Work out the finished part from the listing and answer in its coordinate system (mm). A direction names the side the tool comes from. Coordinates: 2 decimals unless noted, no trailing zeros. Order: outer loops, then holes, each group sorted by start corner. A loop starts at its lowest first (then second) coordinate and runs counter-clockwise, first axis right, second up. Notation, with made-up numbers: M 84.25,78.5 L 140.25,78.5 A25 cw 140.25,90.5 Z; hole C -27,-3.5 d8. An arc over 180 degrees is marked long. Answer in a Markdown table with one row per item. Add a question column.
Item 1: Which of the six approach directions +Z, -Z, +X, -X, +Y, -Y give full straight-line access (tool end or side, diameter ignored) to faces 1 (the face through (69, -44, 0.254)), 2 (the face through (69, -88.9, 8))?
Item 2: The part is cut by section A-A (z = 2.75). Write down the section's boundary in (x, y).
Item 3: Consider line 1 (Z direction, x = 99, y = -11); line 2 (X direction, y = -35.5, z = 4.75); line 3 (X direction, y = -69.5, z = 13). Determine where each line is inside the solid, lowest interval first. Write a range as from..to.
Item 4: The part is cut by section C-C (y = -20.5). Write down the section's boundary in (x, z).
Item 5: Flat-ended cylindrical pins translate along their axes: pin 1 Ø1 at (y, z) = (-40.5, 8) entering from -X; pin 2 Ø1.5 at (y, z) = (-75.5, 12) entering from -X; pin 3 Ø3 at (x, z) = (123, 5) entering from -Y. Find the tip coordinate at first contact, or state that the pin passes through.
Item 6: The mould has two halves that part along X. Classify faces 3 (the face through (69, -88.646, 8)), 4 (the face through (69, -44, 0)): released by +X, released by -X, zero draft, split by the parting line, or undercut.
Item 7: The part is cut by section B-B (x = 47.5). Write down the section's boundary in (y, z).
from build123d import *

# Parameters (mm, degrees)
F1_DEPTH = 16.51
F2_T     = -0.254


with BuildPart() as f1:
    # F0 (on Top) → F1 (new body)
    with BuildSketch(Plane.XY):
        with BuildLine():
            Line((95.25, 0), (44.45, 0))
            ThreePointArc((44.45, 0), (13.019104, -13.019104), (0, -44.45))
            ThreePointArc((0, -44.45), (13.019104, -75.880896), (44.45, -88.9))
            Line((44.45, -88.9), (95.25, -88.9))
            ThreePointArc((95.25, -88.9), (126.680896, -75.880896), (139.7, -44.45))
            ThreePointArc((139.7, -44.45), (126.680896, -13.019104), (95.25, 0))
        make_face()
    extrude(amount=F1_DEPTH)

    # F2
    f2_openings = [f1.faces().sort_by_distance(p)[0] for p in [
        (69.85, -44.45, 16.51),
    ]]
    offset(amount=F2_T, openings=f2_openings)


solid = f1.part
Reply:
| question | item | result |
|---|---|---|
| 1 | face 1 | +Z |
| 1 | face 2 | +Z, -Z, +X, -X, -Y |
| 2 | outline | M 0,-44.45 A44.45 ccw 44.45,-88.9 L 95.25,-88.9 A44.45 ccw 139.7,-44.45 A44.45 ccw 95.25,0 L 44.45,0 A44.45 ccw Z; hole M 0.25,-44.45 A44.2 ccw 44.45,-88.65 L 95.25,-88.65 A44.2 ccw 139.45,-44.45 A44.2 ccw 95.25,-0.25 L 44.45,-0.25 A44.2 ccw Z |
| 3 | line 1 | z = 0..0.25 |
| 3 | line 2 | x = 0.91..1.17, 138.53..138.79 |
| 3 | line 3 | x = 7.73..8.04, 131.66..131.97 |
| 4 | outline | M 7,0 L 132.7,0 L 132.7,16.51 L 132.39,16.51 L 132.39,0.25 L 7.31,0.25 L 7.31,16.51 L 7,16.51 Z |
| 5 | pin 1 | stops at x = 0.13 |
| 5 | pin 2 | stops at x = 11.93 |
| 5 | pin 3 | stops at y = -80.32 |
| 6 | face 3 | undercut |
| 6 | face 4 | zero draft |
| 7 | outline | M -88.9,0 L 0,0 L 0,16.51 L -0.25,16.51 L -0.25,0.25 L -88.65,0.25 L -88.65,16.51 L -88.9,16.51 Z |
